from build123d import *

# Parameters (mm, degrees)
SKETCH1_R           = 52.4
SKETCH1_R_2         = 4.925
SKETCH1_R_3         = 2.9
BOSS_EXTRUDE1_DEPTH = 3


with BuildPart() as part:
    # Sketch1 → Boss-Extrude1 (new body)
    with BuildSketch(Plane(origin=(0, 0, 0), x_dir=(1, 0, 0), z_dir=(0, 1, 0))):
        Circle(SKETCH1_R)
        Circle(SKETCH1_R_2, mode=Mode.SUBTRACT)
        with Locations((0, 34.925)):
            Circle(SKETCH1_R_3, mode=Mode.SUBTRACT)
        with Locations((34.925, 0)):
            Circle(SKETCH1_R_3, mode=Mode.SUBTRACT)
        with Locations((0, -34.925)):
            Circle(SKETCH1_R_3, mode=Mode.SUBTRACT)
        with Locations((-34.925, 0)):
            Circle(SKETCH1_R_3, mode=Mode.SUBTRACT)
    extrude(amount=BOSS_EXTRUDE1_DEPTH)


solid = part.part
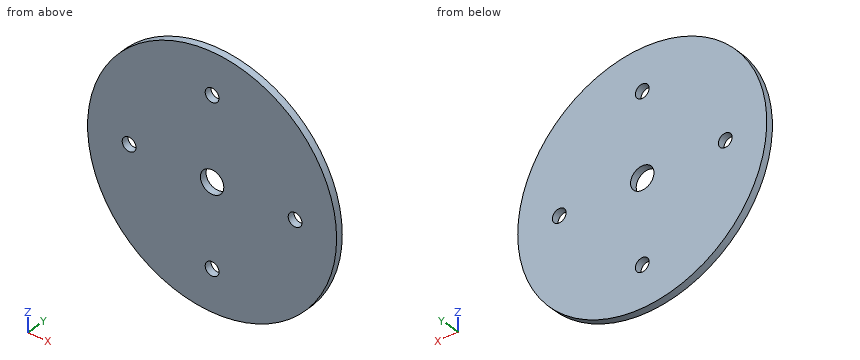
For this review, take the finished solid that the model builds, in its own axes (mm). Give positions to 0.01 mm unless a question says otherwise; leave off trailing zeros. Loops run counter-clockwise (first coordinate to the right, second up) from the corner with the lowest first, then second, coordinate; pieces in that order, holes last. Notation, with made-up numbers: M 44,33.5 L 57,33.5 A18 cw 57,37.5 Z; hole C 3,59 d9. An arc over 180 degrees is marked long. Put each result on its own line as item: value. Start each with the question number.
(1) Add section A-A, the plane x = 0. Write out the cut boundary in (y, z) (3 decimals), then the cut area to 3 significant figures.
(2) For pin 1 (4.5 mm diameter, centred on x = -34.925, z = 0, fed in from -Y); pin 2 (13 mm diameter, centred on x = 0, z = 0, fed in from +Y); pin 3 (1 mm diameter, centred on x = 38, y = 2, fed in from -Z), all flat-tipped, find the tip position at first contact; note any pin that passes through.
(3) Add section C-C, the plane x = -36.5. Write out the cut boundary in (y, z).
(4) Add section D-D, the plane y = 0.6. Write out the cut boundary in (x, z) (3 decimals).
(5) Wall thickness on L1, parallel to X at y = 1.9, z = 0 (3 decimals); L2, parallel to X at y = 1.95, z = -1: over which ranges is each line inside the solid? List them lowest first.
(6) Add section B-B, the plane z = 0. Write out the cut boundary in (x, y) (3 decimals).
Result:
1. outline: M 0,-52.4 L 3,-52.4 L 3,-37.825 L 0,-37.825 Z; M 0,-32.025 L 3,-32.025 L 3,-4.925 L 0,-4.925 Z; M 0,4.925 L 3,4.925 L 3,32.025 L 0,32.025 Z; M 0,37.825 L 3,37.825 L 3,52.4 L 0,52.4 Z
1. area: 250 mm^2
2. pin 1: passes through
2. pin 2: stops at y = 3
2. pin 3: stops at z = -36.6
3. outline: M 0,-37.6 L 3,-37.6 L 3,-2.44 L 0,-2.44 Z; M 0,2.44 L 3,2.44 L 3,37.6 L 0,37.6 Z
4. outline: C 0,0 d104.8; hole C -34.925,0 d5.8; hole C 0,0 d9.85; hole C 0,-34.925 d5.8; hole C 0,34.925 d5.8; hole C 34.925,0 d5.8
5. L1: x = -52.4 to -37.825, -32.025 to -4.925, 4.925 to 32.025, 37.825 to 52.4
5. L2: x = -52.39 to -37.65, -32.2 to -4.82, 4.82 to 32.2, 37.65 to 52.39
6. outline: M -52.4,0 L -37.825,0 L -37.825,3 L -52.4,3 Z; M -32.025,0 L -4.925,0 L -4.925,3 L -32.025,3 Z; M 4.925,0 L 32.025,0 L 32.025,3 L 4.925,3 Z; M 37.825,0 L 52.4,0 L 52.4,3 L 37.825,3 Z
